```python
from build123d import *

# Parameters (mm, degrees)
SKETCH1_W               = 30.48
SKETCH1_H               = 30.48
BOSS_EXTRUDE1_DEPTH     = 19.05
SKETCH4_R               = 9.1
CUT_EXTRUDE1_DEPTH      = 15.24
CUT_EXTRUDE2_REACH      = 30.765
SKETCH5_R               = 2.669997608
CUT_EXTRUDE3_DEPTH      = 29.764869198
CUT_EXTRUDE3_DEPTH_BACK = 19.05
SKETCH6_OUTSIDE_W       = 41.906
SKETCH6_OUTSIDE_H       = 41.906


with BuildPart() as part:
    # Sketch1 → Boss-Extrude1 (new body)
    with BuildSketch(Plane(origin=(0, 0, 0), x_dir=(1, 0, 0), z_dir=(0, 1, 0))):
        Rectangle(SKETCH1_W, SKETCH1_H)
    extrude(amount=BOSS_EXTRUDE1_DEPTH)

    # Sketch4 → Cut-Extrude1 (cut)
    with BuildSketch(Plane(origin=(0, 19.05, 0), x_dir=(1, 0, 0), z_dir=(0, 1, 0))):
        with Locations(Location((0, 0, 0), (0, 0, 270))):
            Circle(SKETCH4_R)
    extrude(amount=-CUT_EXTRUDE1_DEPTH, mode=Mode.SUBTRACT)

    # Sketch5 → Cut-Extrude2 (cut, up to next)
    with BuildSketch(Plane.XZ, mode=Mode.PRIVATE) as cut_extrude2_sk1:
        with Locations(Location((0, 0, 0), (0, 0, 270))):
            Circle(SKETCH5_R)
    cut_extrude2_tool1 = extrude(cut_extrude2_sk1.sketch, amount=-CUT_EXTRUDE2_REACH, mode=Mode.PRIVATE) & part.part
    add(cut_extrude2_tool1.solids().sort_by_distance((0, 0, 0))[0], mode=Mode.SUBTRACT)

    # Sketch6 outside → Cut-Extrude3 (cut, two sides: drawn at the far end of the back side and taken through both)
    with BuildSketch(Plane(origin=(0, 19.05, 0), x_dir=(1, 0, 0), z_dir=(0, 1, 0)).offset(-CUT_EXTRUDE3_DEPTH_BACK)):
        Rectangle(SKETCH6_OUTSIDE_W, SKETCH6_OUTSIDE_H)
        Polygon((-7.62, 15.24), (-7.62, 12.7), (-9.525, 12.7), (-9.525, 10.16), (-3.175, 10.16), (-3.175, 12.7), (-5.08, 12.7), (-5.08, 15.24), (5.08, 15.24), (5.08, 12.7), (3.175, 12.7), (3.175, 10.16), (9.525, 10.16), (9.525, 12.7), (7.62, 12.7), (7.62, 15.24), (10.16, 15.24), (10.16, 7.62), (12.7, 7.62), (12.7, 9.525), (15.24, 9.525), (15.24, 3.175), (12.7, 3.175), (12.7, 5.08), (10.16, 5.08), (10.16, -5.08), (12.7, -5.08), (12.7, -3.175), (15.24, -3.175), (15.24, -9.525), (12.7, -9.525), (12.7, -7.62), (10.16, -7.62), (10.16, -15.24), (7.62, -15.24), (7.62, -12.7), (9.525, -12.7), (9.525, -10.16), (3.175, -10.16), (3.175, -12.7), (5.08, -12.7), (5.08, -15.24), (-5.08, -15.24), (-5.08, -12.7), (-3.175, -12.7), (-3.175, -10.16), (-9.525, -10.16), (-9.525, -12.7), (-7.62, -12.7), (-7.62, -15.24), (-10.16, -15.24), (-10.16, -7.62), (-12.7, -7.62), (-12.7, -9.525), (-15.24, -9.525), (-15.24, -3.175), (-12.7, -3.175), (-12.7, -5.08), (-10.16, -5.08), (-10.16, 5.08), (-12.7, 5.08), (-12.7, 3.175), (-15.24, 3.175), (-15.24, 9.525), (-12.7, 9.525), (-12.7, 7.62), (-10.16, 7.62), (-10.16, 15.24), align=None, mode=Mode.SUBTRACT)
    extrude(amount=CUT_EXTRUDE3_DEPTH + CUT_EXTRUDE3_DEPTH_BACK, mode=Mode.SUBTRACT)


solid = part.part
```
Check sheet for the modelled part. Datum: model origin and axes. Units: mm. A direction names the side the tool comes from. Give positions to 0.01 mm unless a question says otherwise; leave off trailing zeros. Write each loop counter-clockwise with the first axis right and the second up, starting at its lowest first coordinate (ties: lowest second). Pieces come first, ordered by that corner, then holes. Notation, with made-up numbers: (9, 35.25) - (17, 35.25) arc R26 ccw to (17, 49.25) - close; hole circle Ø6 at (35, -21). An arc over 180 degrees is marked (long way). Answer as a JSON object with one key per item and string values. Group by question number.
1) Thickness scan on probe 1 along Z at (x, y) = (4.5, 2); probe 2 along Z at (x, y) = (10.5, 2.25); probe 3 along X at (y, z) = (11.5, 0). Record the ranges inside material, lowest first. Write a range as from..to.
2) Sectioned sample at D-D (x = 8). Record the cut outline in (y, z).
3) Sectioned sample at C-C (z = 0). Record the cut outline in (x, y), then the cut area to 3 significant figures.
4) Sectioned sample at A-A (z = 11.5). Record the cut outline in (x, y) (3 decimals).
5) Access from +Z, -Z, +X, -X, +Y, -Y to the whole of each face (thin tool, end or side, straight path). Record for faces 3 (the face through (6, 9, -10.16)), 4 (the face through (-10.16, 9, 11)), 5 (the face through (-15.24, 9, 6)), 6 (the face through (7.62, 9, -14)), 7 (the face through (15.24, 9, 6)).
6) Release check for a two-part mould opening along Z. For faces 1 (the face through (-7.62, 9, 14)), 2 (the face through (10.16, 9, 0)) record: pulls with the +Z half, pulls with the -Z half, needs draft (parallel to the pull), parting line crosses it, or undercut.
7) Depth check by flat-ended pin: P1, Ø0.8, axis at x = -11.5, y = 7, coming from the -Z side; P2, Ø1.3, axis at x = 14, y = 5.5, coming from the +Z side (3 decimals); P3, Ø4, axis at y = 4.5, z = 1, coming from the -X side. Enter the tip coordinate at first touch or a pass-through.
8) Sectioned sample at B-B (x = 0). Record the cut outline in (y, z), then the cut area to 3 significant figures.
Geometry results:
{
 "1": {"probe 1": "z = -15.24..-12.7, -10.16..10.16, 12.7..15.24", "probe 2": "z = -7.62..-5.08, 5.08..7.62", "probe 3": "x = -10.16..-9.1, 9.1..10.16"},
 "2": {"outline": "(0, -15.24) - (19.05, -15.24) - (19.05, -12.7) - (0, -12.7) - close; (0, -10.16) - (19.05, -10.16) - (19.05, -4.34) - (3.81, -4.34) - (3.81, 4.34) - (19.05, 4.34) - (19.05, 10.16) - (0, 10.16) - close; (0, 12.7) - (19.05, 12.7) - (19.05, 15.24) - (0, 15.24) - close"},
 "3": {"outline": "(-10.16, 0) - (-2.67, 0) - (-2.67, 3.81) - (-9.1, 3.81) - (-9.1, 19.05) - (-10.16, 19.05) - close; (2.67, 0) - (10.16, 0) - (10.16, 19.05) - (9.1, 19.05) - (9.1, 3.81) - (2.67, 3.81) - close", "area": "89.4 mm^2"},
 "4": {"outline": "(-10.16, 0) - (-9.525, 0) - (-9.525, 19.05) - (-10.16, 19.05) - close; (-3.175, 0) - (3.175, 0) - (3.175, 19.05) - (-3.175, 19.05) - close; (9.525, 0) - (10.16, 0) - (10.16, 19.05) - (9.525, 19.05) - close"},
 "5": {"face 3": "+Y, -Y", "face 4": "+Z, +Y, -Y", "face 5": "+Z, -Z, -X, +Y, -Y", "face 6": "-Z, +Y, -Y", "face 7": "+Z, -Z, +X, +Y, -Y"},
 "6": {"face 1": "needs draft", "face 2": "undercut"},
 "7": {"P1": "stops at z = -7.62", "P2": "stops at z = 9.525", "P3": "stops at x = -10.16"},
 "8": {"outline": "(0, -15.24) - (19.05, -15.24) - (19.05, -9.1) - (3.81, -9.1) - (3.81, -2.67) - (0, -2.67) - close; (0, 2.67) - (3.81, 2.67) - (3.81, 9.1) - (19.05, 9.1) - (19.05, 15.24) - (0, 15.24) - close", "area": "283 mm^2"}
}
